Can you work these out from the model? Positions are in its coordinate system, mm. A direction names the side the tool comes from. Round coordinates to 2 decimals unless told otherwise and drop trailing zeros. Write each loop counter-clockwise with the first axis right and the second up, starting at its lowest first coordinate (ties: lowest second). Pieces come first, ordered by that corner, then holes.
Q1. For faces 5 (the flat face through (15, 13, 66)), 6 (the flat face through (8, 10, 38)), 7 (the cylindrical face through (15, 17, 55)), which set-ups out of +Z, -Z, +X, -X, +Y, -Y let a thin tool reach every point of the face, with its end or its side?
Q2. If we section it at A-A (z = 47): Please give me the cut outline in (x, y), plus the area to 3 significant figures.
Q3. Please list where these lines run through material, in increasing order: line 1 along Z through (x, y) = (15, 21.5); line 2 along Z through (x, y) = (18.25, 17.5); line 3 along X through (y, z) = (12, 32).
Q4. If we section it at C-C (y = 20): Please give me the cut outline in (x, z), plus the area to 3 significant figures.
Q5. If we section it at D-D (x = 21.5): Please give me the cut outline in (y, z), plus the area to 3 significant figures.
Q6. We'd pull the mould along Z, two halves only. Please class faces 1 (the cylindrical face through (15, 17, 20)), 2 (the flat face through (20, 17, 37)), 3 (the flat face through (5, 20, 80)), 4 (the flat face through (2.927, 17.395, 14.93)): +Z half, -Z half, draft (parallel to the pull), parting line (faces both ways), or undercut.
Q7. I'm going to push flat-ended pins straight in: pin 1 Ø4 at (y, z) = (18.5, 28) entering from -X; pin 2 Ø8 at (y, z) = (20, 78) entering from +X; pin 3 Ø4 at (x, y) = (4.5, 18) entering from +Z; pin 4 Ø2 at (x, y) = (26, 18.5) entering from +Z. Where does each tip first touch, or does it pass through?
Q8. If we section it at B-B (x = 15): Please give me the cut outline in (y, z).
from build123d import *

# Parameters (mm, degrees)
F1_DEPTH = 30
F2_R     = 5
F3_DEPTH = 15.001
F4_DEPTH = 15.001


with BuildPart() as f1:
    # F0 (on Right) → F1 (new body)
    with BuildSketch(Plane.YZ):
        Polygon((15, 66), (10, 66), (10, 10), (25, 10), (25, 90), (15, 90), align=None)
    extrude(amount=F1_DEPTH)

    # F2 (on face) → F3 (cut, through all)
    with BuildSketch(Plane.XZ.offset(-10)):
        with BuildLine():
            Line((10, 50), (10, 25))
            ThreePointArc((10, 25), (15, 20), (20, 25))
            Line((20, 25), (20, 50))
            ThreePointArc((20, 50), (15, 55), (10, 50))
        make_face()
        with Locations((15, 75)):
            Circle(F2_R)
        Polygon((30, 10), (30, 20), (24.226497, 10), align=None)
        Polygon((5.773503, 10), (0, 20), (0, 10), align=None)
    extrude(amount=-F3_DEPTH, mode=Mode.SUBTRACT)

    # F2 (on face) → F4 (cut, through all)
    with BuildSketch(Plane.XZ.offset(-10)):
        Polygon((0, 70), (10, 90), (0, 90), align=None)
        Polygon((30, 90), (20, 90), (30, 70), align=None)
    extrude(amount=-F4_DEPTH, mode=Mode.SUBTRACT)


solid = f1.part
A:
1. face 5: +Z, +X, -X, -Y
1. face 6: +Z, -Z, +X, -X, -Y
1. face 7: +Y, -Y
2. outline: (0, 10) - (10, 10) - (10, 25) - (0, 25) - close; (20, 10) - (30, 10) - (30, 25) - (20, 25) - close
2. area: 300 mm2
3. line 1: z = 10 to 20, 55 to 70, 80 to 90
3. line 2: z = 10 to 21.2, 53.8 to 71.2, 78.8 to 90
3. line 3: x = 0 to 10, 20 to 30
4. outline: (0, 20) - (5.77, 10) - (24.23, 10) - (30, 20) - (30, 70) - (20, 90) - (10, 90) - (0, 70) - close; hole (10, 25) arc R5 ccw to (20, 25) - (20, 50) arc R5 ccw to (10, 50) - close; hole circle Ø10 at (15, 75)
4. area: 1,740 mm2
5. outline: (10, 10) - (25, 10) - (25, 87) - (15, 87) - (15, 66) - (10, 66) - close
5. area: 1,050 mm2
6. face 1: undercut
6. face 2: undercut
6. face 3: +Z half
6. face 4: -Z half
7. pin 1: stops at x = 0
7. pin 2: stops at x = 28
7. pin 3: stops at z = 83
7. pin 4: stops at z = 80
8. outline: (10, 10) - (25, 10) - (25, 20) - (10, 20) - close; (10, 55) - (25, 55) - (25, 70) - (15, 70) - (15, 66) - (10, 66) - close; (15, 80) - (25, 80) - (25, 90) - (15, 90) - close
